Source: three-view drawing plus pictorial views. Frame: mm from the lowest corner of the part. Round coordinates to 2 decimals unless told otherwise and drop trailing zeros. Order: outer loops, then holes, each group sorted by start corner. A loop starts at its lowest first (then second) coordinate and runs counter-clockwise, first axis right, second up. Notation, with made-up numbers: (63.5, 31.5) - (112.5, 31.5) arc R5 cw to (112.5, 36.5) - close; hole circle Ø7 at (15.5, -35.5). An arc over 180 degrees is marked (long way). One line per item, written item: value. Start each with the question number.
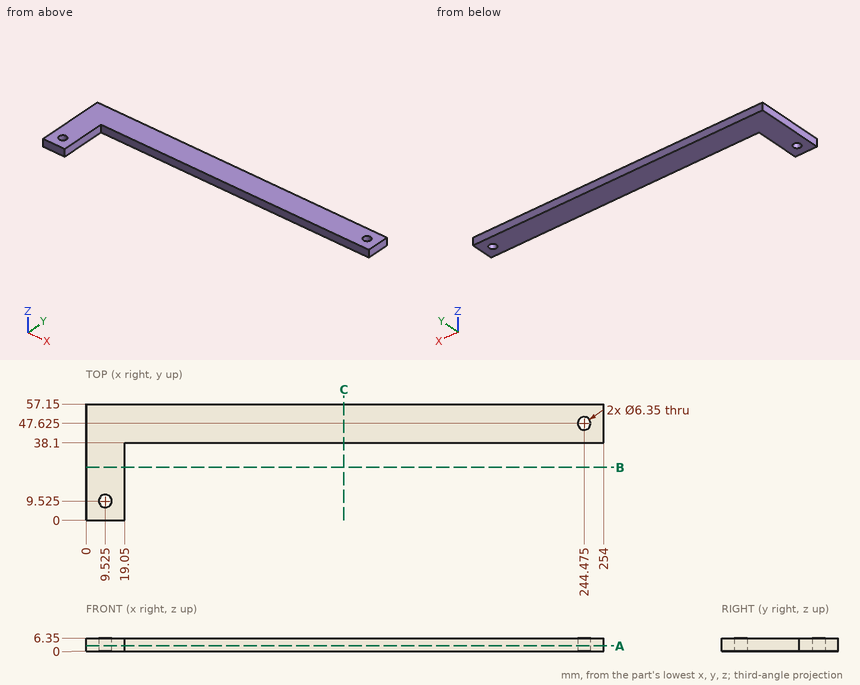
Item 1: Section query A-A on z = 2.75. Return loops of the section in (x, y) (3 decimals), and give its area (3 significant figures).
Item 2: Section query B-B on y = 26. Return loops of the section in (x, z), and give its area (3 significant figures).
Item 3: First-contact query: pin 1 Ø1 at (x, z) = (223, 1.5) entering from -Y; pin 2 Ø7.5 at (x, y) = (244.475, 47.625) entering from -Z. Flat tips, straight axial feed; report the tip coordinate or a pass-through.
Item 4: Line query: L1, parallel to X at y = 9.5, z = 1.25; L2, parallel to Y at x = 227, z = 4.5; L3, parallel to X at y = 13, z = 5.75. Output: solid intervals per line, ascending.
Item 5: Section query C-C on x = 126.5. Return loops of the section in (y, z).
Geometry results:
1. outline: (0, 0) - (19.05, 0) - (19.05, 38.1) - (254, 38.1) - (254, 57.15) - (0, 57.15) - close; hole circle Ø6.35 at (9.525, 9.525); hole circle Ø6.35 at (244.475, 47.625)
1. area: 5,500 mm^2
2. outline: (0, 0) - (19.05, 0) - (19.05, 6.35) - (0, 6.35) - close
2. area: 121 mm^2
3. pin 1: stops at y = 38.1
3. pin 2: stops at z = 0
4. L1: x = 0 to 6.35, 12.7 to 19.05
4. L2: y = 38.1 to 57.15
4. L3: x = 0 to 19.05
5. outline: (38.1, 0) - (57.15, 0) - (57.15, 6.35) - (38.1, 6.35) - close
